Build history of the part. All positions in model axes, mm. Give positions to 0.01 mm unless a question says otherwise; leave off trailing zeros. Loops run counter-clockwise (first coordinate to the right, second up) from the corner with the lowest first, then second, coordinate; pieces in that order, holes last. Notation, with made-up numbers: M -1.5,-24 L 45.5,-24 A20 cw 45.5,8 Z; hole C 58,59.25 d10. An arc over 180 degrees is marked long. Put each result on its own line as item: value.
```python
from build123d import *

# Parameters (mm, degrees)
SKETCH_1_W          = 15
SKETCH_1_H          = 25
EXTRUDE_1_DEPTH     = 15
SKETCH_4_W          = 33.460320445
SKETCH_4_H          = 26.687965621
CUT_EXTRUDE_1_DEPTH = 15
SKETCH_5_W          = 41.021028331
SKETCH_5_H          = 23.23593172
CUT_EXTRUDE_2_DEPTH = 15


with BuildPart() as part:
    # 草圖1 → 填料-伸長1 (new body)
    with BuildSketch(Plane(origin=(0, 0, 0), x_dir=(1, 0, 0), z_dir=(0, 1, 0))):
        Rectangle(SKETCH_1_W, SKETCH_1_H)
    extrude(amount=EXTRUDE_1_DEPTH)

    # 草圖4 → 除料-伸長1 (cut)
    with BuildSketch(Plane(origin=(-9.689922481, 4.84496124, 1.937984496), x_dir=(0.157499846, -0.078749923, 0.984374039), z_dir=(-0.880450906, 0.440225453, 0.176090181))):
        with Locations((1.566467167, 5.33065366)):
            Rectangle(SKETCH_4_W, SKETCH_4_H)
    extrude(amount=CUT_EXTRUDE_1_DEPTH, mode=Mode.SUBTRACT)

    # 草圖5 → 除料-伸長2 (cut)
    with BuildSketch(Plane(origin=(8.101851852, 8.101851852, 3.240740741), x_dir=(-0.19245009, -0.19245009, 0.962250449), z_dir=(-0.680413817, -0.680413817, -0.272165527))):
        with Locations((-1.846019689, 5.465840721)):
            Rectangle(SKETCH_5_W, SKETCH_5_H)
    extrude(amount=-CUT_EXTRUDE_2_DEPTH, mode=Mode.SUBTRACT)


solid = part.part
```
Q1. Slice it at A-A (y = 11). List the corners of the cut face in (x, z).
Here are the results:
outline: M -7.5,-12.5 L 7.5,-12.5 L 7.5,-2.5 L 1.5,12.5 L -4.5,12.5 L -7.5,-2.5 Z
Q2. Slice it at C-C (x = 6). List the corners of the cut face in (y, z).
Here are the results:
outline: M 0,-12.5 L 15,-12.5 L 15,-8.75 L 6.5,12.5 L 0,12.5 Z
Q3. Probe line 1 (Z direction, x = 3, y = 11.5); line 2 (Y direction, x = 5.5, z = 5); line 3 (Y direction, x = -5, z = 7.75). List the from-to ranges inside material, lowest first. Write a range as from..to.
Here are the results:
line 1: -12.5..7.5
line 2: 0..10
line 3: 0..11.9
Q4. Slice it at D-D (x = -4.5). List the corners of the cut face in (y, z).
Here are the results:
outline: M 0,-12.5 L 15,-12.5 L 15,2.5 L 11,12.5 L 0,12.5 Z
Q5. Slice it at B-B (z = -2.5). List the corners of the cut face in (x, y), and give its area (3 significant figures).
Here are the results:
outline: M -7.5,0 L 7.5,0 L 7.5,11 L 3.5,15 L -5.5,15 L -7.5,11 Z
area: 213 mm²
